Source: CAD feature listing. Evaluate the final solid. Frame: model axes, mm. A direction names the side the tool comes from. Round coordinates to 2 decimals unless told otherwise and drop trailing zeros. Loops run counter-clockwise (first coordinate to the right, second up) from the corner with the lowest first, then second, coordinate; pieces in that order, holes last. Notation, with made-up numbers: (17.25, 55.5) -> (71.25, 55.5) arc R24 ccw to (71.25, 78.5) -> close; hole circle Ø8 at (89, 47.25). An arc over 180 degrees is marked (long way). Return JSON: item names as keys, results as strings. Group by question number.
Autodesk Inventor part; units mm, degrees
ref_plane "slider_spacer_sensor_dog_XY" through (0, -10, 47) normal (0, 1, 0) x (1, 0, 0)
ref_plane "slider_spacer_sensor_dog_YZ" through (0, -10, 47) normal (1, 0, 0) x (0, 0, -1)
ref_plane "slider_spacer_sensor_dog_ZX" through (0, -10, 47) normal (0, 0, -1) x (0, 1, 0)
sketch "Sketch_1" plane through (0, 0, 0) normal (1, 0, 0) x (0, 1, 0)
  line L0 (22, 52) -> (-8.5, 52)
  arc A0 (-8.5, 52) -> (-10, 50.5) centre (-8.5, 50.5) ccw
  line L1 (-10, 50.5) -> (-10, 26.75)
  line L2 (-10, 26.75) -> (0, 26.75)
  line L3 (0, 26.75) -> (0, -26.75)
  line L4 (0, -26.75) -> (-10, -26.75)
  line L5 (-10, -26.75) -> (-10, -50.5)
  arc A1 (-10, -50.5) -> (-8.5, -52) centre (-8.5, -50.5) ccw
  line L6 (-8.5, -52) -> (22, -52)
  line L7 (22, -52) -> (22, -40)
  line L8 (22, -40) -> (0, -40)
  arc A2 (-1, -39) -> (0, -40) centre (0, -39) ccw
  line L9 (-1, -39) -> (-1, -35)
  arc A3 (0, -34) -> (-1, -35) centre (0, -35) ccw
  line L10 (0, -34) -> (7, -34)
  arc A4 (7, -34) -> (10, -31) centre (7, -31) ccw
  line L11 (10, -31) -> (10, 31)
  arc A5 (10, 31) -> (7, 34) centre (7, 31) ccw
  line L12 (7, 34) -> (0, 34)
  arc A6 (-1, 35) -> (0, 34) centre (0, 35) ccw
  line L13 (-1, 35) -> (-1, 39)
  arc A7 (0, 40) -> (-1, 39) centre (0, 39) ccw
  line L14 (0, 40) -> (22, 40)
  line L15 (22, 40) -> (22, 52)
extrude "Extrusion1" add sketch "Sketch_1" along normal mid plane 81
sketch "Sketch2" plane through (-40.5, 22, 40) normal (0, 1, 0) x (1, 0, 0)
  point P0 (17.5, -6)
hole "Drilling 1" at (-23, 22, 46) direction (0, -1, 0) diameter 4.917 depth 13.5 tip angle 140 countersink diameter 6 countersink angle 90
pattern_linear "Rectangular Pattern1" count 2 spacing 46 along (1, 0, 0) count 2 spacing 92 along (0, 0, -1) of "Drilling 1"
sketch "Sketch3" plane through (-40.5, -10, 50.5) normal (0, -1, 0) x (1, 0, 0)
  point P0 (38, -3.5)
hole "Drilling 2" at (-2.5, -10, 47) direction (0, 1, 0) diameter 2.1129 depth 6 tip angle 140 countersink diameter 2.6 countersink angle 90
pattern_linear "Rectangular Pattern2" count 2 spacing 5 along (1, 0, 0) count 2 spacing 94 along (0, 0, -1) of "Drilling 2"
ref_plane "slider_spacer_sensor_dog_XY" through (0, -10, 47) normal (0, 1, 0) x (1, 0, 0)
ref_plane "slider_spacer_sensor_dog_YZ" through (0, -10, 47) normal (1, 0, 0) x (0, 0, -1)
ref_plane "slider_spacer_sensor_dog_ZX" through (0, -10, 47) normal (0, 0, -1) x (0, 1, 0)
ref_plane "slider_spacer_slider_XY" through (0, 0, 0) normal (0, 1, 0) x (1, 0, 0)
ref_plane "slider_spacer_slider_YZ" through (0, 0, 0) normal (1, 0, 0) x (0, 0, -1)
ref_plane "slider_spacer_slider_ZX" through (0, 0, 0) normal (0, 0, -1) x (0, 1, 0)
properties part number "KR45H-A-Slider Spacer"
(1) Mould query, pull axis Z, two halves, no side actions, for faces 1 (the face through (2.52, -3.64, 46.94)), 2 (the face through (40.5, 6, 1)), 3 (the face through (-1, 7, 52)). Classes: released by +Z, released by -Z, zero draft, split by the parting line, or undercut.
(2) Cut plane D-D (z = -3.5). Return loops of the section in (x, y).
(3) Cut plane A-A (y = -7). Return loops of the section in (x, z), and give its area (3 significant figures).
(4) Cut plane C-C (z = 28). Return loops of the section in (x, y).
(5) Set-up query: faces 4 (the face through (-22.06, 14.89, -43.73)), 5 (the face through (-2.817, -6.838, -48.008)), 6 (the face through (-1, 10, 0)), 7 (the face through (-1, -10, 39)). Return all of +Z, -Z, +X, -X, +Y, -Y with unobstructed straight access to the full face (end or side cutting, diameter ignored); none if empty.
(6) Cut plane B-B (x = 14). Return loops of the section in (y, z), and give its area (3 significant figures).
(7) Ray query, line 1 (Z direction, x = 2.5, y = -8.1); line 2 (X direction, y = 12.5, z = -46); line 3 (X direction, y = -7, z = 47). Return the intervals inside material, ascending.
(8) Pin query (flat end, axial travel): pin 1 (8 mm diameter, centred on x = 16, z = -10, fed in from -Y); pin 2 (2.5 mm diameter, centred on x = -2.5, z = -47, fed in from -Y); pin 3 (1.2 mm diameter, centred on x = -1.5, z = 37, fed in from +Y); pin 4 (5 mm diameter, centred on y = -3, z = 15, fed in from +X). Return the tip coordinate at first contact, or that it passes through.
Answers follow:
{
 "1": {"face 1": "undercut", "face 2": "zero draft", "face 3": "released by +Z"},
 "2": {"outline": "(-40.5, 0) -> (40.5, 0) -> (40.5, 10) -> (-40.5, 10) -> close"},
 "3": {"outline": "(-40.5, -52) -> (40.5, -52) -> (40.5, -26.75) -> (-40.5, -26.75) -> close; (-40.5, 26.75) -> (40.5, 26.75) -> (40.5, 52) -> (-40.5, 52) -> close; hole circle Ø2.11 at (-2.5, -47); hole circle Ø2.11 at (-2.5, 47); hole circle Ø2.11 at (2.5, -47); hole circle Ø2.11 at (2.5, 47)", "area": "4,080 mm^2"},
 "4": {"outline": "(-40.5, -10) -> (40.5, -10) -> (40.5, 10) -> (-40.5, 10) -> close"},
 "5": {"face 4": "+Y", "face 5": "-Y", "face 6": "+X, -X, +Y", "face 7": "+Z, -Z, +X, -X, -Y"},
 "6": {"outline": "(-10, -50.5) arc R1.5 ccw to (-8.5, -52) -> (22, -52) -> (22, -40) -> (0, -40) arc R1 cw to (-1, -39) -> (-1, -35) arc R1 cw to (0, -34) -> (7, -34) arc R3 ccw to (10, -31) -> (10, 31) arc R3 ccw to (7, 34) -> (0, 34) arc R1 cw to (-1, 35) -> (-1, 39) arc R1 cw to (0, 40) -> (22, 40) -> (22, 52) -> (-8.5, 52) arc R1.5 ccw to (-10, 50.5) -> (-10, 26.75) -> (0, 26.75) -> (0, -26.75) -> (-10, -26.75) -> close", "area": "1,700 mm^2"},
 "7": {"line 1": "-52 to -48.06, -45.94 to -26.75, 26.75 to 45.94, 48.06 to 52", "line 2": "-40.5 to -25.46, -20.54 to 20.54, 25.46 to 40.5", "line 3": "-40.5 to -3.56, -1.44 to 1.44, 3.56 to 40.5"},
 "8": {"pin 1": "y = 0", "pin 2": "y = -9.95", "pin 3": "y = -1", "pin 4": "through"}
}
